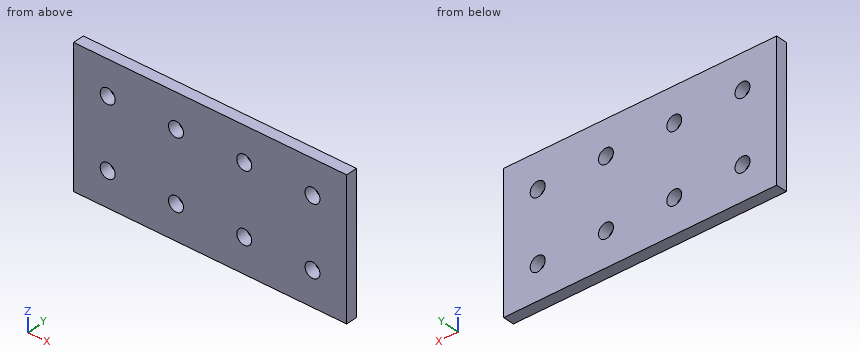
```python
from build123d import *

# Parameters (mm, degrees)
SKETCH1_W                        = 152.4
SKETCH1_H                        = 76.2
BOSS_EXTRUDE1_DEPTH              = 6.35
F_21_64_0_32813_DIAMETER_HOLE1_D = 8.334502
LPATTERN1_COUNT                  = 2
LPATTERN1_PITCH                  = 38.1
LPATTERN1_COUNT_DIR2             = 4
LPATTERN1_PITCH_DIR2             = 38.1


with BuildPart() as part:
    # Sketch1 → Boss-Extrude1 (new body)
    with BuildSketch(Plane(origin=(0, 0, 0), x_dir=(1, 0, 0), z_dir=(0, 1, 0))):
        with Locations((76.2, 38.1)):
            Rectangle(SKETCH1_W, SKETCH1_H)
    extrude(amount=BOSS_EXTRUDE1_DEPTH)

    # 21/64 (0.32813) Diameter Hole1 (through all)
    with Locations(Plane(origin=(0, 6.35, 0), x_dir=(1, 0, 0), z_dir=(0, 1, 0))):
        with Locations((19.05, 57.15)):
            f_21_64_0_32813_diameter_hole1 = Hole(F_21_64_0_32813_DIAMETER_HOLE1_D / 2)

    # LPattern1: 21_64 _0.32813_ Diameter Hole1 2 × 4
    with Locations(*[(j * LPATTERN1_PITCH_DIR2, 0, i * LPATTERN1_PITCH) for i in range(LPATTERN1_COUNT) for j in range(LPATTERN1_COUNT_DIR2) if (i, j) != (0, 0)]):
        add(f_21_64_0_32813_diameter_hole1, mode=Mode.SUBTRACT)


solid = part.part
```
Verification items for the finished model (mm, model axes). Give positions to 0.01 mm unless a question says otherwise; leave off trailing zeros. Order: outer loops, then holes, each group sorted by start corner. A loop starts at its lowest first (then second) coordinate and runs counter-clockwise, first axis right, second up. Notation, with made-up numbers: (89, -18) -> (111, -18) arc R13 ccw to (111, -4) -> close; hole circle Ø6 at (34.25, 83.25). An arc over 180 degrees is marked (long way). Use a Markdown table: item, result.
1) Section check B-B, the plane x = 55.5. Record the boundary of the cut face in (y, z).
Results:
| item | result |
|---|---|
| outline | (0, -76.2) -> (6.35, -76.2) -> (6.35, -60.98) -> (0, -60.98) -> close; (0, -53.32) -> (6.35, -53.32) -> (6.35, -22.88) -> (0, -22.88) -> close; (0, -15.22) -> (6.35, -15.22) -> (6.35, 0) -> (0, 0) -> close |
2) Material ranges on probe 1 along X at (y, z) = (1.5, -57.15); probe 2 along Z at (x, y) = (133.35, 2.75); probe 3 along Z at (x, y) = (135, 4.75), recorded low to high.
Results:
| item | result |
|---|---|
| probe 1 | 0 to 14.88, 23.22 to 52.98, 61.32 to 91.08, 99.42 to 129.18, 137.52 to 152.4 |
| probe 2 | -76.2 to -61.32, -52.98 to -23.22, -14.88 to 0 |
| probe 3 | -76.2 to -60.98, -53.32 to -22.88, -15.22 to 0 |
3) Depth check by flat-ended pin: pin 1 Ø5 at (x, z) = (133.35, -57.15) entering from -Y. Enter the tip coordinate at first touch or a pass-through.
Results:
| item | result |
|---|---|
| pin 1 | through |
4) Section check A-A, the plane y = 4. Give the number of separate pieces and of enclosed holes in the cut face, then the cut area to 3 significant figures.
Results:
| item | result |
|---|---|
| separate pieces | 1 |
| enclosed holes | 8 |
| area | 11,200 mm² |
5) Section check C-C, the plane z = -19.05. Record the boundary of the cut face in (x, y).
Results:
| item | result |
|---|---|
| outline | (0, 0) -> (14.88, 0) -> (14.88, 6.35) -> (0, 6.35) -> close; (23.22, 0) -> (52.98, 0) -> (52.98, 6.35) -> (23.22, 6.35) -> close; (61.32, 0) -> (91.08, 0) -> (91.08, 6.35) -> (61.32, 6.35) -> close; (99.42, 0) -> (129.18, 0) -> (129.18, 6.35) -> (99.42, 6.35) -> close; (137.52, 0) -> (152.4, 0) -> (152.4, 6.35) -> (137.52, 6.35) -> close |
